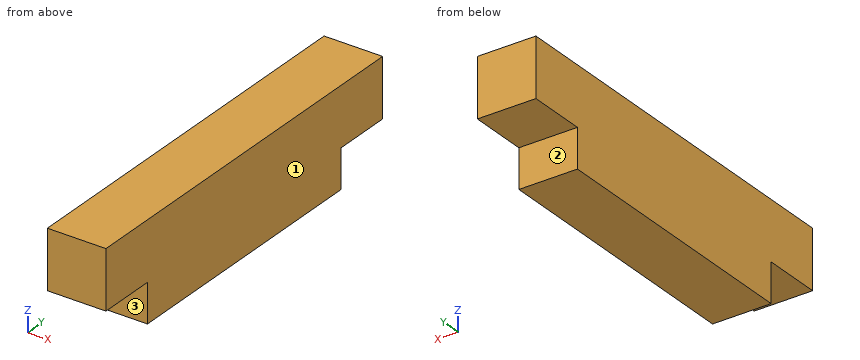
from build123d import *

# Parameters (mm, degrees)
F0_W     = 15
F0_H     = 15
F1_DEPTH = 50
F0_H_2   = 10
F2_DEPTH = 35


with BuildPart() as f1:
    # F0 (on Front) → F1 (new body, symmetric)
    with BuildSketch(Plane.XZ):
        with Locations((-0.108219, -2.080006)):
            Rectangle(F0_W, F0_H)
    extrude(amount=F1_DEPTH, both=True)

    # F0 (on Front) → F2 (join, symmetric)
    with BuildSketch(Plane.XZ):
        with Locations((-0.108219, -14.580006)):
            Rectangle(F0_W, F0_H_2)
    extrude(amount=F2_DEPTH, both=True)


solid = f1.part
Geometry: final body of the model. Coordinates: model frame, mm. Face numbers are marked on the shaded views. A direction names the side the tool comes from. Give positions to 0.01 mm unless a question says otherwise; leave off trailing zeros. Order: outer loops, then holes, each group sorted by start corner. A loop starts at its lowest first (then second) coordinate and runs counter-clockwise, first axis right, second up. Notation, with made-up numbers: (85, -28.75) -> (144, -28.75) arc R20 ccw to (144, -17.75) -> close; hole circle Ø8 at (-25.75, 37). An arc over 180 degrees is marked (long way). Put each result on its own line as item: value.
Q1. Section C-C, the plane z = -14.75. Return loops of the section in (x, y).
Here are the results:
outline: (-7.61, -35) -> (7.39, -35) -> (7.39, 35) -> (-7.61, 35) -> close
Q2. Pin query (flat end, axial travel): pin 1 (5 mm diameter, centred on x = 0, z = -16, fed in from -Y); pin 2 (5 mm diameter, centred on x = -3.5, z = -13.5, fed in from +Y); pin 3 (4.5 mm diameter, centred on x = 2.5, y = 43.5, fed in from -Z). Return the tip coordinate at first contact, or that it passes through.
Here are the results:
pin 1: stops at y = -35
pin 2: stops at y = 35
pin 3: stops at z = -9.58
Q3. Reachability of the marked faces 1, 2 and 3 from +Z, -Z, +X, -X, +Y, -Y: full face, straight path, thin tool, end or side. Return the list, or none.
Here are the results:
face 1: +Z, -Z, +X, +Y, -Y
face 2: -Z, +X, -X, +Y
face 3: -Z, +X, -X, -Y
Q4. Section A-A, the plane x = 4.25. Return loops of the section in (y, z).
Here are the results:
outline: (-50, -9.58) -> (-35, -9.58) -> (-35, -19.58) -> (35, -19.58) -> (35, -9.58) -> (50, -9.58) -> (50, 5.42) -> (-50, 5.42) -> close
Q5. Section B-B, the plane y = -38. Return loops of the section in (x, z), then the cut area to 3 significant figures.
Here are the results:
outline: (-7.61, -9.58) -> (7.39, -9.58) -> (7.39, 5.42) -> (-7.61, 5.42) -> close
area: 225 mm^2
Q6. Material intervals for L1, parallel to Y at x = 2.5, z = -13.5; L2, parallel to Z at x = 6.25, y = 41, sorted ascending.
Here are the results:
L1: y = -35 to 35
L2: z = -9.58 to 5.42
